```python
from build123d import *

# Parameters (mm, degrees)
F0_R     = 37.5
F1_DEPTH = 20
F2_W     = 37
F2_H     = 37
F3_DEPTH = 37
F4_W     = 25
F4_H     = 25


with BuildPart() as f1:
    # F0 (on Front) → F1 (new body)
    with BuildSketch(Plane.XZ):
        Circle(F0_R)
    extrude(amount=-F1_DEPTH)

    # F2 (on face) → F3 (join)
    with BuildSketch(Plane(origin=(0, 20, 0), x_dir=(-1, 0, 0), z_dir=(0, 1, 0))):
        Rectangle(F2_W, F2_H)
    extrude(amount=F3_DEPTH)

    # F4 (on face) → F8 section 0
    with BuildSketch(Plane(origin=(0, 57, 0), x_dir=(-1, 0, 0), z_dir=(0, 1, 0)), mode=Mode.PRIVATE) as f8_s0:
        Rectangle(F4_W, F4_H)
    loft([f8_s0.sketch, Vertex(0, 94, 0)])


solid = f1.part
```
Check sheet for the modelled part. Datum: model origin and axes. Units: mm. A direction names the side the tool comes from. Round coordinates to 2 decimals unless told otherwise and drop trailing zeros. Order: outer loops, then holes, each group sorted by start corner. A loop starts at its lowest first (then second) coordinate and runs counter-clockwise, first axis right, second up. Notation, with made-up numbers: (18, 39) -> (43, 39) arc R25 ccw to (43, 73) -> close; hole circle Ø2 at (-9.75, 86.5). An arc over 180 degrees is marked (long way). One line per item, written item: value. Start each with the question number.
Q1. Set-up check for faces 1 (the face through (18.5, 38, 0)), 2 (the face through (-18.5, 38, 0)), 3 (the face through (13, 57, 0)), 4 (the face through (0, 38, 18.5)), 5 (the face through (0, 38, -18.5)): record each of +Z, -Z, +X, -X, +Y, -Y from which the full face is reachable in a straight line by a thin tool's end or side.
Q2. Cross-section at C-C (y = 18.5). Record the boundary of the cut face in (x, z).
Q3. Gauge pin test, flat ends, axial feed: pin 1 Ø11 at (x, y) = (0, 32) entering from -Z; pin 2 Ø10 at (x, z) = (20, 13) entering from +Y; pin 3 Ø18.5 at (x, y) = (-3.5, 35) entering from +Z. Record the tip position at first contact, or that the pin passes through.
Q4. Cross-section at A-A (y = 53.5). Record the boundary of the cut face in (x, z).
Q5. Thickness scan on line 1 (X direction, y = 5, z = 1); line 2 (X direction, y = 28, z = -10.5); line 3 (Y direction, x = -22, z = 26). Record the ranges inside material, lowest first.
Q6. Cross-section at D-D (x = 29.5). Record the boundary of the cut face in (y, z).
Q7. Cross-section at B-B (x = -7). Record the boundary of the cut face in (y, z).
Completed:
1. face 1: +Z, -Z, +X, +Y
1. face 2: +Z, -Z, -X, +Y
1. face 3: +Y
1. face 4: +Z, +X, -X, +Y
1. face 5: -Z, +X, -X, +Y
2. outline: circle Ø75 at (0, 0)
3. pin 1: stops at z = -18.5
3. pin 2: stops at y = 57
3. pin 3: stops at z = 18.5
4. outline: (-18.5, -18.5) -> (18.5, -18.5) -> (18.5, 18.5) -> (-18.5, 18.5) -> close
5. line 1: x = -37.49 to 37.49
5. line 2: x = -18.5 to 18.5
5. line 3: y = 0 to 20
6. outline: (0, -23.15) -> (20, -23.15) -> (20, 23.15) -> (0, 23.15) -> close
7. outline: (0, -36.84) -> (20, -36.84) -> (20, -18.5) -> (57, -18.5) -> (57, -12.5) -> (73.28, -7) -> (73.28, 7) -> (57, 12.5) -> (57, 18.5) -> (20, 18.5) -> (20, 36.84) -> (0, 36.84) -> close
